from build123d import *

# Parameters (mm, degrees)
ESQUISSE1_W             = 30
ESQUISSE1_H             = 10
ESQUISSE3_W             = 32
ESQUISSE3_H             = 12
ENL_V_MAT_EXTRU_1_DEPTH = 34.166247904


with BuildPart() as part:
    # Esquisse1 → Révolution2 (revolve)
    with BuildSketch(Plane.XY, mode=Mode.PRIVATE) as r_volution2_sk:
        with Locations((15, 5)):
            Rectangle(ESQUISSE1_W, ESQUISSE1_H)
    revolve(r_volution2_sk.sketch.rotate(Axis((0, 0, 0), (1, 0, 0)), 90), axis=Axis((0, 0, 0), (1, 0, 0)))

    # Esquisse2 → Chambrage pour vis à tête hexagonale M81 (revolve, cut)
    with BuildSketch(Plane(origin=(30, 0, 0), x_dir=(0, 0, -1), z_dir=(0, 1, 0))):
        Polygon((0, 0), (0, 22.703872786), (4.5, 20), (4.5, 10.04330127), (4.525, 10), (7.5, 10), (7.5, 0), align=None)
    revolve(axis=Axis((36.35, 0, 0), (-1, 0, 0)), mode=Mode.SUBTRACT)

    # Esquisse3 → Enlèv. mat.-Extru.1 (cut, through all)
    with BuildSketch(Plane(origin=(30, 0, 0), x_dir=(0, 0, -1), z_dir=(1, 0, 0))):
        with Locations((-0.50912904, 6)):
            Rectangle(ESQUISSE3_W, ESQUISSE3_H)
    extrude(amount=-ENL_V_MAT_EXTRU_1_DEPTH, mode=Mode.SUBTRACT)


solid = part.part
Build history of the part. All positions in model axes, mm. A direction names the side the tool comes from. Coordinates: 2 decimals unless noted, no trailing zeros. Write each loop counter-clockwise with the first axis right and the second up, starting at its lowest first coordinate (ties: lowest second). Pieces come first, ordered by that corner, then holes. Notation, with made-up numbers: (55, -3) -> (78, -3) arc R27 cw to (78, 28) -> close; hole circle Ø9 at (20, -2). An arc over 180 degrees is marked (long way). Use CSV: the item, a comma, the result in double quotes. Start each with the question number.
Q1. Drill centre lines: probe 1 along X at (y, z) = (-2.75, -4.5); probe 2 along Z at (x, y) = (24, -6.75); probe 3 along Z at (x, y) = (23.5, -2.25). Where is each one in solid material? Low to high.
Q2. Cut at A-A, the plane z = 0. List the corners of the cut face in (x, y) (3 decimals), then the cut area to 3 significant figures.
Q3. Pull direction Z, two halves, no side cores. Call faces 1 (the cylindrical face through (15, -10, 0)), 2 (the cylindrical face through (25.07, -7.5, -0.16)), 3 (the flat face through (0, -4, 0)), 4 (the flat face through (20, -5, 0)): released by +Z, released by -Z, zero draft, split by the parting line, or undercut.
Q4. Cut at C-C, the plane x = 10.75. List the corners of the cut face in (y, z), then the cut area to 3 significant figures.
Q5. Cut at B-B, the plane y = -8. List the corners of the cut face in (x, z), then the cut area to 3 significant figures.
Q6. Flat gauge pins, fed straight in: pin 1 Ø3 at (x, y) = (3, -2) entering from +Z; pin 2 Ø3 at (x, z) = (11, 1.5) entering from +Y; pin 3 Ø6 at (x, z) = (25, 2) entering from +Y. Where does each tip first touch, or does it go through?
Q7. Cut at D-D, the plane z = 5. List the corners of the cut face in (x, y).
Q8. 3-axis set-ups, long thin cutter, end or side, ignore diameter. For faces 5 (the cylindrical face through (15, -4.5, -0.1)), 6 (the flat face through (8.5, 0, 2.4)): which of +Z, -Z, +X, -X, +Y, -Y reach the whole face in a straight line?
Checked values:
1,probe 1,"x = 0 to 20"
1,probe 2,"z = -7.38 to -3.27, 3.27 to 7.38"
1,probe 3,"z = -9.74 to -7.15, 7.15 to 9.74"
2,outline,"(0, -10) -> (30, -10) -> (30, -7.5) -> (20, -7.5) -> (20, -4.525) -> (19.957, -4.5) -> (10, -4.5) -> (7.296, 0) -> (0, 0) -> close"
2,area,"174 mm²"
3,face 1,"split by the parting line"
3,face 2,"undercut"
3,face 3,"zero draft"
3,face 4,"undercut"
4,outline,"(0, -10) -> (0, -4.5) arc R4.5 cw to (0, 4.5) -> (0, 10) arc R10 ccw to start"
4,area,"125 mm²"
5,outline,"(0, -6) -> (30, -6) -> (30, 6) -> (0, 6) -> close"
5,area,"360 mm²"
6,pin 1,"stops at z = 9.99"
6,pin 2,"stops at y = -3.24"
6,pin 3,"stops at y = -5.59"
7,outline,"(0, -8.66) -> (30, -8.66) -> (30, -5.59) -> (20, -5.59) -> (20, 0) -> (0, 0) -> close"
8,face 5,"+X, +Y"
8,face 6,"+Z, -Z, +X, -X, +Y"
